Build history of the part. All positions in model axes, mm. Round coordinates to 2 decimals unless told otherwise and drop trailing zeros. Write each loop counter-clockwise with the first axis right and the second up, starting at its lowest first coordinate (ties: lowest second). Pieces come first, ordered by that corner, then holes.
1) Wall check: probe 1 along Y at (x, z) = (0, -8); probe 2 along Y at (x, z) = (0, 291); probe 3 along X at (y, z) = (283.5, 11.5). Give the ranges that are in metal, low to high.
2) Saw through at C-C (z = 293.5). Write the cut outline in (x, y), plus the area to 3 significant figures.
3) Flat gauge pins, fed straight in: pin 1 (4 mm diameter, centred on x = -258.5, z = 193.5, fed in from -Y); pin 2 (5 mm diameter, centred on y = 299, z = 144.5, fed in from -X); pin 3 (1 mm diameter, centred on x = -112, z = 254.5, fed in from +Y). Where does each tip first touch, or does it go through?
4) Saw through at D-D (z = 72). Write the cut outline in (x, y), plus the area to 3 significant figures.
Autodesk Inventor part; units mm, degrees
ref_plane "YZ Plane" through (0, 0, 0) normal (1, 0, 0) x (0, 1, 0)
ref_plane "XZ Plane" through (0, 0, 0) normal (0, 1, 0) x (-1, 0, 0)
ref_plane "XY Plane" through (0, 0, 0) normal (0, 0, 1) x (1, 0, 0)
sketch "Sketch1" plane through (0, 0, 0) normal (0, 0, 1) x (1, 0, 0)
  circle A0 centre (0, 0) radius 361.95
  circle A1 centre (0, 0) radius 393.7
  dimension "d0" = 723.9
  dimension "d1" = 787.4
extrude "Extrusion1" add sketch "Sketch1" along normal blind 304.8
sketch "Sketch2" plane through (0, 0, 304.8) normal (0, 0, 1) x (1, 0, 0)
  circle A0 centre (0, 0) radius 393.7
  circle A1 centre (0, 0) radius 396.621
  circle A2 centre (0, 0) radius 399.796
  dimension "d4" = 793.242
  dimension "d5" = 799.592
extrude "Extrusion2" add sketch "Sketch2" against normal blind 50.8 contours A1
extrude "Extrusion3" add sketch "Sketch2" against normal blind 25.4 contours A2
chamfer "Chamfer1" distance 2.921 angle 45 1 edges at (-393.7, 0, 254)
sketch "Sketch3" plane through (0, 0, 0) normal (0, 0, -1) x (-1, 0, 0)
  circle A0 centre (0, 0) radius 380.746
  circle A1 centre (0, 0) radius 361.95
  dimension "d13" = 761.492
extrude "Extrusion4" add sketch "Sketch3" along normal blind 12.7
fillet "Fillet1" radius 0.7937 2 edges at (380.746, 0, 0) (-396.621, 0, 279.4)
chamfer "Chamfer2" distance 0.7937 angle 45 1 edges at (380.746, 0, -12.7)
chamfer "Chamfer3" distance 0.7937 angle 45 1 edges at (-399.796, 0, 279.4)
sketch "Sketch4" plane through (0, 0, 0) normal (1, 0, 0) x (0, 1, 0)
  line L0 (396.621, 278.6062) -> (396.621, 254) construction
  line L1 (-399.796, 304.8) -> (399.796, 304.8) construction
  line L2 (396.621, 273.05) -> (394.8409, 271.2699)
  arc A0 (394.8409, 271.2699) -> (393.446, 267.9023) centre (398.2085, 267.9023) ccw
  line L3 (393.446, 267.9023) -> (393.446, 267.0852)
  arc A1 (393.446, 267.0852) -> (394.8409, 263.7176) centre (398.2085, 267.0852) ccw
  line L4 (394.8409, 263.7176) -> (396.621, 261.9375)
  line L5 (396.621, 261.9375) -> (396.621, 273.05)
  line L6 (0, -60.96) -> (0, 365.76)
  point P0 (0, 0)
  dimension "d23" = 11.1125
  dimension "d24" = 3.175
  dimension "d25" = 4.7625
  dimension "d26" = 31.75
  dimension "d27" = 45
revolve "Revolution1" cut sketch "Sketch4" angle 360 about axis through (0, 0, -10) along (0, 0, 1)
sketch "Sketch7" plane through (0, 0, -12.7) normal (0, 0, -1) x (-1, 0, 0)
  circle A0 centre (0, 0) radius 361.95
  circle A1 centre (0, 0) radius 393.7
extrude "Extrusion7" add sketch "Sketch7" along normal mid plane 25.4
sketch "Sketch8" plane through (0, 0, 304.8) normal (0, 0, 1) x (1, 0, 0)
  circle A0 centre (0, 0) radius 399.796
  circle A1 centre (0, 0) radius 361.95
  circle A2 centre (0, 0) radius 406.146
  dimension "d43" = 6.35
extrude "Extrusion8" add sketch "Sketch8" along normal blind 12.7 and the other way blind 50.8 contours A0 | A2
chamfer "Chamfer4" distance 9.525 angle 45 1 edges at (-406.146, 0, 254)
equation "\"d10\" = -0.5 * d1 + 0.5 * d4"
properties part number "A1-19037-200-06 HCWI liner - pup - as cast" material "Iron, HCWI"
Evaluation:
1. probe 1: y = -393.7 to -361.95, 361.95 to 393.7
1. probe 2: y = -406.15 to -361.95, 361.95 to 406.15
1. probe 3: x = -273.18 to -225.02, 225.02 to 273.18
2. outline: circle Ø812.29 at (0, 0); hole circle Ø723.9 at (0, 0)
2. area: 107,000 mm2
3. pin 1: stops at y = -298.68
3. pin 2: stops at x = -259.01
3. pin 3: stops at y = 381.54
4. outline: circle Ø787.4 at (0, 0); hole circle Ø723.9 at (0, 0)
4. area: 75,400 mm2
